Solid Edge part; units mm, degrees
sketch "Sketch1" plane through (0, 0, 0) normal (0, 0, 1) x (1, 0, 0)
  line L0 (-6.5, 0) -> (-6.5, -8)
  line L1 (-6.5, -8) -> (6.5, -8)
  line L2 (6.5, -8) -> (6.5, 0)
  line L3 (6.5, 0) -> (7.5, 0)
  line L4 (7.5, 0) -> (7.5, 12)
  line L5 (7.5, 12) -> (5, 12)
  line L6 (5, 12) -> (5, 2)
  line L7 (5, 2) -> (-5, 2)
  line L8 (-5, 2) -> (-5, 12)
  line L9 (-5, 12) -> (-7.5, 12)
  line L10 (-7.5, 12) -> (-7.5, 0)
  line L11 (-7.5, 0) -> (-6.5, 0)
  dimension "D1" = 6.5
  dimension "D2" = 6.5
  dimension "D3" = 5
  dimension "D4" = 5
  dimension "D5" = 5
  dimension "D6" = 7.5
extrude "Ajout_matière_1" add sketch "Sketch1" along normal mid plane 100
hole "Perçage_1" at (0, -8, 42) direction (0, 1, 0) diameter 4.459 end up to next
pattern_linear "Pattern1" count 7 spacing 14 along (0, 0, -1) of "Perçage_1"
sketch "Sketch2" plane through (0, 2, -50) normal (0, 0, -1) x (0, 1, 0)
  line L0 (-10, -6.5) -> (-2, -6.5)
  line L1 (-2, -6.5) -> (-2, -7.5)
  line L2 (-2, -7.5) -> (10, -7.5)
  line L3 (10, -7.5) -> (10, 7.5)
  line L4 (10, 7.5) -> (-2, 7.5)
  line L5 (-2, 7.5) -> (-2, 6.5)
  line L6 (-2, 6.5) -> (-10, 6.5)
  line L7 (-10, 6.5) -> (-10, -6.5)
extrude "Protrusion1" add sketch "Sketch2" along normal mid plane 2.5
mirror "Mirror1" about plane through (0, 0, 0) normal (0, 0, 1) of "Protrusion1"
hole "Perçage_2" at (0, 7, 51.25) direction (0, 0, -1) diameter 5 end through all
chamfer "Chamfer1" distance 1 angle 45 4 edges at (-7.5, 12, 0) (-6.5, 0, 0) (6.5, 0, 0) (7.5, 12, 0)
properties material "Aluminium AU4G, 2024_T4"
The listing builds one solid part. Answer for the finished solid, in the listing's coordinates (mm). A direction names the side the tool comes from. Round coordinates to 2 decimals unless told otherwise and drop trailing zeros. Write each loop counter-clockwise with the first axis right and the second up, starting at its lowest first coordinate (ties: lowest second). Pieces come first, ordered by that corner, then holes. Notation, with made-up numbers: (-17, 4) -> (20, 4) arc R27 ccw to (20, 23) -> close; hole circle Ø6 at (83.5, -11.75). An arc over 180 degrees is marked (long way). Use CSV: the item, a comma, the result in double quotes. Start each with the question number.
(1) Section C-C on x = 0 is taken. Count the separate pieces of the cut face and the enclosed holes in it, then the cut area to 3 significant figures.
(2) Each of these flat-tipped pins is pushed along its axis until it touches: pin 1 (6 mm diameter, centred on x = 0, z = -14, fed in from +Y); pin 2 (5.5 mm diameter, centred on y = -5, z = -21, fed in from +X); pin 3 (3.5 mm diameter, centred on y = -4.5, z = -12, fed in from -X). Where does it stop, or does it pass through?
(3) Consider L1, parallel to Y at x = 0, z = 50.45; L2, parallel to X at y = 2.25, z = -12.5; L3, parallel to X at y = -5.5, z = 28. Determine where each line is inside the solid, lowest interval first. Write a range as from..to.
(4) The mould has two halves that part along X. Classify faces 4 (the face through (0.098, -3.07, 16.227)), 5 (the face through (-3, -8, -1)), 6 (the face through (6.5, -5, -1)): released by +X, released by -X, zero draft, split by the parting line, or undercut.
(5) Section D-D on y = -7 is taken. Give the vertices of the cut face in (x, z), then the cut area to 3 significant figures.
(6) Section B-B on y = 8 is taken. Give the vertices of the cut face in (x, z), then the cut area to 3 significant figures.
(7) Which of the six approach directions +Z, -Z, +X, -X, +Y, -Y give full straight-line access (tool end or side, diameter ignored) to faces 1 (the face through (1.88, -3.07, -43.2)), 2 (the face through (2.3, 2, -0.7)), 3 (the face through (-6.5, -4, -1))?
A:
1,separate pieces,"10"
1,enclosed holes,"0"
1,area,"738 mm²"
2,pin 1,"stops at y = 2"
2,pin 2,"stops at x = 6.5"
2,pin 3,"stops at x = -6.5"
3,L1,"y = -8..4.5, 9.5..12"
3,L2,"x = -7.5..-5, 5..7.5"
3,L3,"x = -6.5..-2.23, 2.23..6.5"
4,face 4,"undercut"
4,face 5,"zero draft"
4,face 6,"released by +X"
5,outline,"(-6.5, -51.25) -> (6.5, -51.25) -> (6.5, 51.25) -> (-6.5, 51.25) -> close; hole circle Ø4.46 at (0, -42); hole circle Ø4.46 at (0, -28); hole circle Ø4.46 at (0, -14); hole circle Ø4.46 at (0, 0); hole circle Ø4.46 at (0, 14); hole circle Ø4.46 at (0, 28); hole circle Ø4.46 at (0, 42)"
5,area,"1,220 mm²"
6,outline,"(-7.5, -51.25) -> (-2.29, -51.25) -> (-2.29, -48.75) -> (-5, -48.75) -> (-5, 48.75) -> (-2.29, 48.75) -> (-2.29, 51.25) -> (-7.5, 51.25) -> close; (2.29, -51.25) -> (7.5, -51.25) -> (7.5, 51.25) -> (2.29, 51.25) -> (2.29, 48.75) -> (5, 48.75) -> (5, -48.75) -> (2.29, -48.75) -> close"
6,area,"540 mm²"
7,face 1,"+Y, -Y"
7,face 2,"+Y"
7,face 3,"+Z, -Z, -X, -Y"
